Geometry check sheet. Reference: the model listing, model coordinates, mm. A direction names the side the tool comes from. Round coordinates to 2 decimals unless told otherwise and drop trailing zeros. Loops run counter-clockwise (first coordinate to the right, second up) from the corner with the lowest first, then second, coordinate; pieces in that order, holes last.
Autodesk Inventor part; units mm, degrees
ref_plane "YZ Plane" through (0, 0, 0) normal (1, 0, 0) x (0, 1, 0)
ref_plane "XZ Plane" through (0, 0, 0) normal (0, 1, 0) x (-1, 0, 0)
ref_plane "XY Plane" through (0, 0, 0) normal (0, 0, 1) x (1, 0, 0)
sketch "Sketch1" plane through (0, 0, 0) normal (0, 0, 1) x (1, 0, 0)
  line L0 (-21.125, 21.125) -> (21.125, 21.125)
  line L1 (21.125, 21.125) -> (21.125, -21.125)
  line L2 (21.125, -21.125) -> (-21.125, -21.125)
  line L3 (-21.125, -21.125) -> (-21.125, 21.125)
  line L4 (-21.125, 21.125) -> (21.125, -21.125) construction
  line L5 (21.125, 21.125) -> (-21.125, -21.125) construction
  point P0 (0, 0)
  dimension "d0" = 42.25
  dimension "d1" = 42.25
extrude "Extrusion1" add sketch "Sketch1" along normal mid plane 47.18
sketch "Sketch2" plane through (0, 0, 23.59) normal (0, 0, 1) x (1, 0, 0)
  circle A0 centre (0, 0) radius 11
  dimension "d4" = 22
extrude "Extrusion2" add sketch "Sketch2" along normal blind 1.97
fillet "Fillet1" radius 3.175 4 edges at (-21.125, 21.125, 0) (-21.125, -21.125, 0) (21.125, 21.125, 0) (21.125, -21.125, 0)
sketch "Sketch3" plane through (0, 0, 25.56) normal (0, 0, 1) x (1, 0, 0)
  circle A0 centre (0, 0) radius 2.5
  dimension "d8" = 5
extrude "Extrusion3" add sketch "Sketch3" along normal blind 22.15
sketch "Sketch4" plane through (0, 0, -23.59) normal (0, 0, -1) x (-1, 0, 0)
  circle A0 centre (-15.76, 15.76) radius 2.95
  circle A1 centre (15.76, 15.76) radius 2.95
  circle A2 centre (-15.76, -15.76) radius 2.95
  circle A3 centre (15.76, -15.76) radius 2.95
  line L0 (-21.125, 17.95) -> (-21.125, -17.95)
  line L1 (17.95, 21.125) -> (-17.95, 21.125)
  line L2 (21.125, -17.95) -> (21.125, 17.95)
  line L3 (-17.95, -21.125) -> (17.95, -21.125)
  point P0 (0, 0)
  dimension "d12" = 5.9
  dimension "d13" = 5.9
  dimension "d14" = 5.9
  dimension "d16" = 5.365
  dimension "d17" = 5.365
  dimension "d18" = 5.365
  dimension "d19" = 5.365
hole "Hole1" at (15.76, 15.76, -23.59) at (-15.76, 15.76, -23.59) at (-15.76, -15.76, -23.59) at (15.76, -15.76, -23.59) direction (0, 0, 1) diameter 5.9 depth 2.2
sketch "Sketch7" plane through (15.76, -15.76, -21.39) normal (0, 0, -1) x (-1, 0, 0)
  circle A0 centre (0, 0) radius 1.524
  point P0 (15.76, 15.76)
  dimension "d46" = 3.048
hole "Hole3" at (15.76, -15.76, -21.39) direction (0, 0, 1) diameter 2.8194 end through all
sketch "Sketch8" plane through (15.76, 15.76, -21.39) normal (0, 0, -1) x (-1, 0, 0)
  circle A0 centre (0, 0) radius 1.524
  point P0 (15.76, -15.76)
  dimension "d54" = 3.048
hole "Hole4" at (15.76, 15.76, -21.39) direction (0, 0, 1) diameter 2.8194 end through all
sketch "Sketch9" plane through (-15.76, -15.76, -21.39) normal (0, 0, -1) x (-1, 0, 0)
  circle A0 centre (0, 0) radius 1.524
  point P0 (-15.76, 15.76)
  dimension "d62" = 3.048
hole "Hole5" at (-15.76, -15.76, -21.39) direction (0, 0, 1) diameter 2.8194 end through all
sketch "Sketch10" plane through (-15.76, 15.76, -21.39) normal (0, 0, -1) x (-1, 0, 0)
  circle A0 centre (0, 0) radius 1.524
  point P0 (-15.76, -15.76)
  dimension "d70" = 3.048
hole "Hole6" at (-15.76, 15.76, -21.39) direction (0, 0, 1) diameter 2.8194 end through all
equation "\"d1\" = d0"
properties part number "CNC- Stepper Motor"
1) Access from +Z, -Z, +X, -X, +Y, -Y to the whole of each face (thin tool, end or side, straight path). Record for faces 1 (the face through (-10, 10, 23.59)), 2 (the face through (-14.902, -16.879, 1.415)), 3 (the face through (13.766, 13.586, -22.475)).
Report:
face 1: +Z
face 2: +Z, -Z
face 3: -Z
2) Scan lines: line 1 along Y through (x, z) = (15.76, -22.1) (3 decimals); line 2 along X through (y, z) = (-15.76, 12.5) (3 decimals). Record each from-to range of solid material in increasing order.
Report:
line 1: y = -21.125 to -18.71, -12.81 to 12.81, 18.71 to 21.125
line 2: x = -21.125 to -17.17, -14.35 to 14.35, 17.17 to 21.125
3) Sectioned sample at D-D, the plane y = 0. Record the cut outline in (x, z) (3 decimals), then the cut area to 3 significant figures.
Report:
outline: (-21.125, -23.59) - (21.125, -23.59) - (21.125, 23.59) - (11, 23.59) - (11, 25.56) - (2.5, 25.56) - (2.5, 47.71) - (-2.5, 47.71) - (-2.5, 25.56) - (-11, 25.56) - (-11, 23.59) - (-21.125, 23.59) - close
area: 2,150 mm2
4) Mould release check, pull along X, two halves, no side actions. Record for faces 4 (the face through (0, -21.125, 0)), 5 (the face through (-2.38, 10.74, 24.56)), 6 (the face through (15.7, -17.17, 1.41)): +X half, -X half, draft (parallel to the pull), parting line (faces both ways), or undercut.
Report:
face 4: draft
face 5: parting line
face 6: undercut
5) Sectioned sample at C-C, the plane z = 19.5. Record the cut outline in (x, y) (3 decimals).
Report:
outline: (-21.125, -17.95) arc R3.175 ccw to (-17.95, -21.125) - (17.95, -21.125) arc R3.175 ccw to (21.125, -17.95) - (21.125, 17.95) arc R3.175 ccw to (17.95, 21.125) - (-17.95, 21.125) arc R3.175 ccw to (-21.125, 17.95) - close; hole circle Ø2.819 at (-15.76, -15.76); hole circle Ø2.819 at (-15.76, 15.76); hole circle Ø2.819 at (15.76, -15.76); hole circle Ø2.819 at (15.76, 15.76)
6) Sectioned sample at A-A, the plane x = 15.76. Record the cut outline in (y, z) (3 decimals), then the cut area to 3 significant figures.
Report:
outline: (-21.125, -23.59) - (-18.71, -23.59) - (-18.71, -21.39) - (-17.17, -21.39) - (-17.17, 23.59) - (-21.125, 23.59) - close; (-14.35, -21.39) - (-12.81, -21.39) - (-12.81, -23.59) - (12.81, -23.59) - (12.81, -21.39) - (14.35, -21.39) - (14.35, 23.59) - (-14.35, 23.59) - close; (17.17, -21.39) - (18.71, -21.39) - (18.71, -23.59) - (21.125, -23.59) - (21.125, 23.59) - (17.17, 23.59) - close
area: 1,710 mm2
7) Gauge pin test, flat ends, axial feed: pin 1 (2 mm diameter, centred on x = -7, z = 28.5, fed in from -Y); pin 2 (5.5 mm diameter, centred on x = -15.76, y = 15.76, fed in from -Z); pin 3 (3.5 mm diameter, centred on x = 15.76, y = 15.76, fed in from +Z). Record the tip position at first contact, or that the pin passes through.
Report:
pin 1: passes through
pin 2: stops at z = -21.39
pin 3: stops at z = 23.59
